Geometry check sheet. Reference: the model listing, model coordinates, mm. A direction names the side the tool comes from. Give positions to 0.01 mm unless a question says otherwise; leave off trailing zeros. Order: outer loops, then holes, each group sorted by start corner. A loop starts at its lowest first (then second) coordinate and runs counter-clockwise, first axis right, second up. Notation, with made-up numbers: M 36,53 L 41,53 A7 ccw 41,62 Z; hole C -17,66.25 d11. An arc over 180 degrees is marked long. Put each result on its own line as item: value. Start each with the question number.
Q1. Access from +Z, -Z, +X, -X, +Y, -Y to the whole of each face (thin tool, end or side, straight path). Record for faces 4 (the cylindrical face through (-30.55, 7.42, -23.43)), 5 (the cylindrical face through (-20.633, 2.535, 15.821)).
Q2. Section check C-C on x = 30.5. Record the cut outline in (y, z), then the cut area to 3 significant figures.
Q3. Section check D-D on z = -31. Record the cut outline in (x, y), then the cut area to 3 significant figures.
Q4. Section check B-B on z = 0. Record the cut outline in (x, y), then the cut area to 3 significant figures.
Q5. Mould release check, pull along Z, two halves, no side actions. Record for faces 1 (the flat face through (8, 9.906, 37)), 2 (the cylindrical face through (-4.88, 7.49, -37.18)), 3 (the cylindrical face through (-21.438, 2.465, -33.625)): +Z half, -Z half, draft (parallel to the pull), parting line (faces both ways), or undercut.
Q6. Go/stop test with flat-tipped pins: pin 1 (3 mm diameter, centred on y = 8.5, z = -24, fed in from -X); pin 2 (5 mm diameter, centred on x = -10.5, y = 2.5, fed in from +Z); pin 3 (3 mm diameter, centred on x = 11.5, y = 8.5, fed in from -Z). Record where each tip stops, or that it passes through.
Q7. Section check A-A on x = 0. Record the cut outline in (y, z), then the cut area to 3 significant figures.
Q8. Material ranges on L1, parallel to Z at x = 0, y = 8.6; L2, parallel to Z at x = -0.5, y = 4.25, recorded low to high.
Autodesk Inventor part; units mm, degrees
ref_plane "YZ Plane" through (0, 0, 0) normal (1, 0, 0) x (0, 1, 0)
ref_plane "XZ Plane" through (0, 0, 0) normal (0, 1, 0) x (-1, 0, 0)
ref_plane "XY Plane" through (0, 0, 0) normal (0, 0, 1) x (1, 0, 0)
sketch "Sketch1" plane through (0, 0, 0) normal (0, 1, 0) x (-1, 0, 0)
  circle A0 centre (0, 0) radius 39.878
  dimension "d0" = 79.756
extrude "Extrusion1" add sketch "Sketch1" along normal blind 5
sketch "Sketch2" plane through (0, 5, 0) normal (0, 1, 0) x (1, 0, 0)
  circle A0 centre (0, 0) radius 26
  dimension "d3" = 52
extrude "Extrusion2" cut sketch "Sketch2" against normal blind 5
thread "Thread1"
sketch "Sketch3" plane through (0, 5, 0) normal (0, 1, 0) x (1, 0, 0)
  circle A0 centre (0, 0) radius 38.5
  dimension "d8" = 77
extrude "Extrusion3" add sketch "Sketch3" along normal blind 4.906
sketch "Sketch4" plane through (0, 9.906, 0) normal (0, 1, 0) x (1, 0, 0)
  circle A0 centre (0, 0) radius 37.5
  dimension "d11" = 75
extrude "Extrusion4" cut sketch "Sketch4" against normal blind 4.906
thread "Thread3"
properties part number "77mm to 52mm" material "Aluminum 6061-AHC"
Results found:
1. face 4: +Y
1. face 5: +Y, -Y
2. outline: M 0,-25.69 L 5,-25.69 L 5,-23.49 L 9.91,-23.49 L 9.91,-21.82 L 5,-21.82 L 5,21.82 L 9.91,21.82 L 9.91,23.49 L 5,23.49 L 5,25.69 L 0,25.69 Z
2. area: 273 mm^2
3. outline: M -25.08,0 L 25.08,0 L 25.08,5 L 22.83,5 L 22.83,9.91 L 21.1,9.91 L 21.1,5 L -21.1,5 L -21.1,9.91 L -22.83,9.91 L -22.83,5 L -25.08,5 Z
3. area: 268 mm^2
4. outline: M -39.88,0 L -26,0 L -26,5 L -37.5,5 L -37.5,9.91 L -38.5,9.91 L -38.5,5 L -39.88,5 Z; M 26,0 L 39.88,0 L 39.88,5 L 38.5,5 L 38.5,9.91 L 37.5,9.91 L 37.5,5 L 26,5 Z
4. area: 149 mm^2
5. face 1: draft
5. face 2: undercut
5. face 3: parting line
6. pin 1: stops at x = -31.24
6. pin 2: stops at z = 39.07
6. pin 3: stops at z = -37.18
7. outline: M 0,-39.88 L 5,-39.88 L 5,-38.5 L 9.91,-38.5 L 9.91,-37.5 L 5,-37.5 L 5,-26 L 0,-26 Z; M 0,26 L 5,26 L 5,37.5 L 9.91,37.5 L 9.91,38.5 L 5,38.5 L 5,39.88 L 0,39.88 Z
7. area: 149 mm^2
8. L1: z = -38.5 to -37.5, 37.5 to 38.5
8. L2: z = -39.87 to -26, 26 to 39.87
